Part print with two shaded views. Sizes in mm from the minimum x, y, z corner. Coordinates: 2 decimals unless noted, no trailing zeros. Write each loop counter-clockwise with the first axis right and the second up, starting at its lowest first coordinate (ties: lowest second). Pieces come first, ordered by that corner, then holes. Notation, with made-up numbers: M 87,-1 L 142,-1 A15 cw 142,27 Z; hole C 88.25,51.5 d11. An arc over 180 degrees is marked long. One line per question, with ' | ' between items. Start each with the question number.
(1) Flat gauge pin, fed straight in: pin 1 Ø5.5 at (x, y) = (1518, 92) entering from -Z. Where does the tip first touch, or does it go through?
(2) Cut at C-C (y = 43). Write the cut outline in (x, z).
(3) Cut at A-A (x = 1266). Write the cut outline in (y, z), plus the area to 3 significant figures.
(4) Cut at B-B (z = 671). Write the cut outline in (x, y).
(5) Wall check: probe 1 along Z at (x, y) = (762, 142); probe 2 along X at (y, z) = (7.5, 450.85); probe 3 along Y at (x, z) = (760, 1424). Give the ranges that are in metal, low to high.
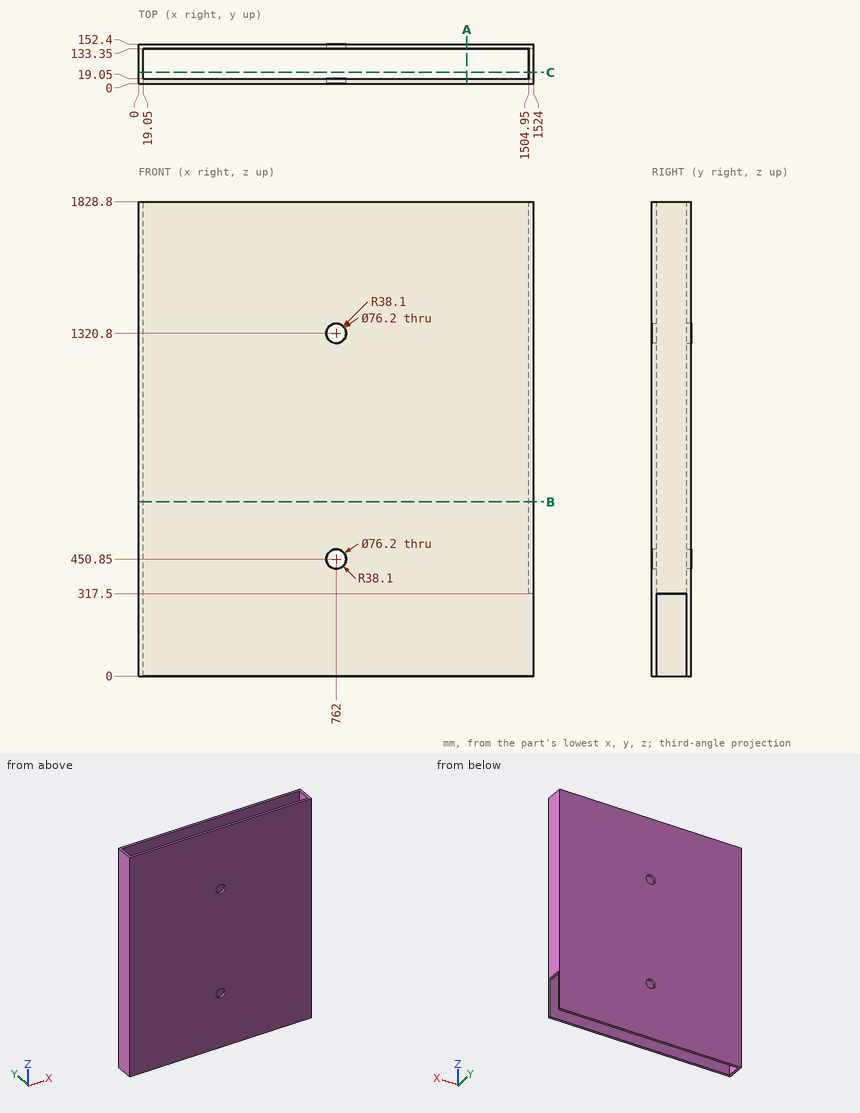
Filled in:
1) pin 1: z = 317.5
2) outline: M 0,0 L 19.05,0 L 19.05,1828.8 L 0,1828.8 Z; M 1504.95,317.5 L 1524,317.5 L 1524,1828.8 L 1504.95,1828.8 Z
3) outline: M 0,0 L 19.05,0 L 19.05,1828.8 L 0,1828.8 Z; M 133.35,0 L 152.4,0 L 152.4,1828.8 L 133.35,1828.8 Z | area: 69,700 mm²
4) outline: M 0,0 L 1524,0 L 1524,152.4 L 0,152.4 Z; hole M 19.05,19.05 L 1504.95,19.05 L 1504.95,133.35 L 19.05,133.35 Z
5) probe 1: 0 to 412.75, 488.95 to 1282.7, 1358.9 to 1828.8 | probe 2: 0 to 723.9, 800.1 to 1524 | probe 3: 0 to 19.05, 133.35 to 152.4
